Autodesk Fusion 360 part; units mm, degrees
sketch "Sketch1" plane through (0, 0, 0) normal (0, 1, 0) x (1, 0, 0)
  line L0 (5, 6.5) -> (-5, 6.5)
  line L1 (-5, 6.5) -> (-5, -6.5)
  line L2 (-5, -6.5) -> (5, -6.5)
  line L3 (5, -6.5) -> (5, 6.5)
  line L4 (5, 6.5) -> (-5, -6.5) construction
  line L5 (-5, 6.5) -> (5, -6.5) construction
  circle A0 centre (0, -1.25) radius 1.5
  dimension "d1" = 13
  dimension "d2" = 10
  dimension "d21" = 3
  dimension "d22" = 1.25
extrude "Extrude1" add sketch "Sketch1" along normal blind 2.5
sketch "Sketch3" plane through (0, 0, 0) normal (0, 1, 0) x (1, 0, 0)
  line L0 (-5, 5) -> (5, 5)
  line L1 (5, 5) -> (5, 7.5)
  line L2 (5, 7.5) -> (-5, 7.5)
  line L3 (-5, 7.5) -> (-5, 5)
  dimension "d10" = 2.5
  dimension "d11" = 10
  dimension "d12" = 5
  dimension "d13" = 5
extrude "Extrude3" add sketch "Sketch3" along normal blind 15
sketch "Sketch5" plane through (0, 0, -5) normal (0, 0, 1) x (1, 0, 0)
  line L0 (5, 2.5) -> (5, 15)
  line L1 (5, 15) -> (-5, 15)
  line L2 (-5, 15) -> (-5, 2.5)
  circle A0 centre (0, 10) radius 1.5
  line L3 (-5, 2.5) -> (5, 2.5)
  dimension "d16" = 5
  dimension "d17" = 3
extrude "Extrude4" cut sketch "Sketch5" against normal blind 45 contours A0
fillet "Fillet1" radius 1.5 2 edges at (0, 2.5, -5) (0, 0, -7.5)
Model file for the job. Use its own axes, mm. A direction names the side the tool comes from. Coordinates: 2 decimals unless noted, no trailing zeros. Loops run counter-clockwise (first coordinate to the right, second up) from the corner with the lowest first, then second, coordinate; pieces in that order, holes last. Notation, with made-up numbers: (14, -6.75) -> (30, -6.75) arc R25 ccw to (30, 17.25) -> close; hole circle Ø8 at (37.25, 72.5). An arc over 180 degrees is marked (long way). Use one line per item in the form item = value. Start each with the question number.
(1) Pull direction Z, two halves, no side cores. Call faces 1 (the cylindrical face through (-0.07, 0.45, -7.07)), 2 (the flat face through (-5, 4.1, -5.3)), 3 (the cylindrical face through (-1.11, 1.23, 2.26)), 4 (the flat face through (0, 8, -5)): pulls with the +Z half, pulls with the -Z half, needs draft (parallel to the pull), parting line crosses it, or undercut.
(2) Cut at A-A on x = 0. Give the cut face in (y, z).
(3) Cut at C-C on y = 10. Give the cut face in (x, z), and give its area (3 significant figures).
(4) Cut at D-D on x = 4.25. Give the cut face in (y, z), and give its area (4 significant figures).
(5) Cut at B-B on z = 1.25. Give the cut face in (x, y), and give its area (3 significant figures).
(6) Flat gauge pins, fed straight in: pin 1 (5 mm diameter, centred on x = 2, y = 12, fed in from +Z); pin 2 (8 mm diameter, centred on y = 7, z = 2, fed in from -X); pin 3 (5 mm diameter, centred on x = -1.5, z = 1.5, fed in from +Y). Where does each tip first touch, or does it go through?
(7) Probe probe 1 along Y at (x, z) = (0, -5.8); probe 2 along X at (y, z) = (1.1, 1.25); probe 3 along Z at (x, y) = (0, 1.85). List the from-to ranges inside material, lowest first. Write a range as from..to.
(8) Tool access for faces 5 (the flat face through (-1, 2.5, 3)), 6 (the cylindrical face through (-0.325, 8.536, -6.232)): list every direction of +Z, -Z, +X, -X, +Y, -Y with a clear straight run to the whole face (end or side of a thin tool).
Values:
q1.face_1 = pulls with the -Z half
q1.face_2 = needs draft
q1.face_3 = undercut
q1.face_4 = pulls with the +Z half
q2.outline = (0, -6) arc R1.5 ccw to (1.5, -7.5) -> (8.5, -7.5) -> (8.5, -5) -> (4, -5) arc R1.5 cw to (2.5, -3.5) -> (2.5, -0.25) -> (0, -0.25) -> close; (0, 2.75) -> (2.5, 2.75) -> (2.5, 6.5) -> (0, 6.5) -> close; (11.5, -7.5) -> (15, -7.5) -> (15, -5) -> (11.5, -5) -> close
q3.outline = (-5, -7.5) -> (-1.5, -7.5) -> (-1.5, -5) -> (-5, -5) -> close; (1.5, -7.5) -> (5, -7.5) -> (5, -5) -> (1.5, -5) -> close
q3.area = 17.5 mm2
q4.outline = (0, -6) arc R1.5 ccw to (1.5, -7.5) -> (15, -7.5) -> (15, -5) -> (4, -5) arc R1.5 cw to (2.5, -3.5) -> (2.5, 6.5) -> (0, 6.5) -> close
q4.area = 66.25 mm2
q5.outline = (-5, 0) -> (-1.5, 0) -> (-1.5, 2.5) -> (-5, 2.5) -> close; (1.5, 0) -> (5, 0) -> (5, 2.5) -> (1.5, 2.5) -> close
q5.area = 17.5 mm2
q6.pin_1 = -5
q6.pin_2 = through
q6.pin_3 = 2.5
q7.probe_1 = 0..8.5, 11.5..15
q7.probe_2 = -5..-1.5, 1.5..5
q7.probe_3 = -7.5..-0.25, 2.75..6.5
q8.face_5 = +Z, +X, -X, +Y
q8.face_6 = +Z, -Z
